Work out the finished part from the listing and answer in its coordinate system (mm). A direction names the side the tool comes from. Coordinates: 2 decimals unless noted, no trailing zeros. Order: outer loops, then holes, each group sorted by start corner. A loop starts at its lowest first (then second) coordinate and runs counter-clockwise, first axis right, second up.
1. Find the intervals of material crossed by probe 1 along X at (y, z) = (-26, 60); probe 2 along Z at (x, y) = (-82.5, -55.5); probe 3 along Y at (x, z) = (65.5, 79), in increasing order.
2. Determine the mould class of faces 1 (the flat face through (-13, -58, 88)), 2 (the cylindrical face through (-155.15, -47.633, 41.658)), 3 (the cylindrical face through (149.726, -44.75, 43.384)) for opening direction X: +X half, -X half, draft (parallel to the pull), parting line (faces both ways), or undercut.
3. A tool of negligible diameter and unlimited length cuts with its end or side. For faces 4 (the flat face through (-2, 2, -6)), 5 (the flat face through (-2, -58, 10)), 6 (the cylindrical face through (-150.2, -44.2, 43.4)), from which of +Z, -Z, +X, -X, +Y, -Y can it reach the whole face along a straight path? Write none if from no direction.
4. Flat-ended cylindrical pins translate along their axes: pin 1 Ø3 at (y, z) = (-57.5, 34) entering from -X; pin 2 Ø5 at (y, z) = (35, 49.5) entering from -X; pin 3 Ø3 at (y, z) = (-57, 53) entering from +X. Find the tip coordinate at first contact, or state that the pin passes through.
5. The part is cut by section A-A, the plane x = 71. Give the vertices of the cut face in (y, z).
6. The part is cut by section D-D, the plane y = 36. Give the vertices of the cut face in (x, z), then the cut area to 3 significant figures.
7. The part is cut by section C-C, the plane y = -30. Give the vertices of the cut face in (x, z).
8. The part is cut by section B-B, the plane z = 82.5. Give the vertices of the cut face in (x, y), then the cut area to 3 significant figures.
```python
from build123d import *

# Parameters (mm, degrees)
BOSS_EXTRUDE1_DEPTH = 88
SKETCH3_W           = 233.89900304
SKETCH3_H           = 68
CUT_EXTRUDE1_DEPTH  = 15
BOSS_EXTRUDE2_DEPTH = 6


with BuildPart() as part:
    # Sketch1 → Boss-Extrude1 (new body)
    with BuildSketch(Plane.XY):
        with BuildLine():
            Line((118.214818276, 64.136748505), (-118.214818276, 64.136748505))
            Line((-118.214818276, 64.136748505), (-162.822637659, -18.216148816))
            ThreePointArc((-162.822637659, -18.216148816), (-154.866072847, -47.976045164), (-126.94950152, -61))
            Line((-126.94950152, -61), (126.94950152, -61))
            ThreePointArc((126.94950152, -61), (154.866072847, -47.976045164), (162.822637659, -18.216148816))
            Line((162.822637659, -18.216148816), (118.214818276, 64.136748505))
        make_face()
        with BuildLine():
            Line((114.641146244, 58.136748505), (-114.641146244, 58.136748505))
            Line((-114.641146244, 58.136748505), (-157.062609578, -20.179799188))
            ThreePointArc((-157.062609578, -20.179799188), (-149.967134226, -44.474777247), (-126.94950152, -55))
            Line((-126.94950152, -55), (126.94950152, -55))
            ThreePointArc((126.94950152, -55), (149.967134226, -44.474777247), (157.062609578, -20.179799188))
            Line((157.062609578, -20.179799188), (114.641146244, 58.136748505))
        make_face(mode=Mode.SUBTRACT)
    extrude(amount=BOSS_EXTRUDE1_DEPTH)

    # Sketch3 → Cut-Extrude1 (cut)
    with BuildSketch(Plane.XZ.offset(46)):
        with Locations((0, 44)):
            Rectangle(SKETCH3_W, SKETCH3_H)
    extrude(amount=CUT_EXTRUDE1_DEPTH, mode=Mode.SUBTRACT)

    # Sketch1<12> → Boss-Extrude2 (add)
    with BuildSketch(Plane.XY):
        with BuildLine():
            Line((162.822637659, -18.216148816), (118.214818276, 64.136748505))
            Line((118.214818276, 64.136748505), (-118.214818276, 64.136748505))
            Line((-118.214818276, 64.136748505), (-162.822637659, -18.216148816))
            ThreePointArc((-162.822637659, -18.216148816), (-154.866072847, -47.976045164), (-126.94950152, -61))
            Line((-126.94950152, -61), (126.94950152, -61))
            ThreePointArc((126.94950152, -61), (154.866072847, -47.976045164), (162.822637659, -18.216148816))
        make_face()
    extrude(amount=-BOSS_EXTRUDE2_DEPTH)


solid = part.part
```
Geometry says:
1. probe 1: x = -163.35 to -157.35, 157.35 to 163.35
1. probe 2: z = -6 to 10, 78 to 88
1. probe 3: y = -61 to -55, 58.14 to 64.14
2. face 1: draft
2. face 2: -X half
2. face 3: undercut
3. face 4: -Z, +X, -X, +Y, -Y
3. face 5: -Y
3. face 6: +Z
4. pin 1: stops at x = -145.37
4. pin 2: stops at x = -135.35
4. pin 3: stops at x = 146.2
5. outline: (-61, -6) - (64.14, -6) - (64.14, 88) - (58.14, 88) - (58.14, 0) - (-55, 0) - (-55, 10) - (-61, 10) - close; (-61, 78) - (-55, 78) - (-55, 88) - (-61, 88) - close
6. outline: (-133.46, -6) - (133.46, -6) - (133.46, 88) - (126.63, 88) - (126.63, 0) - (-126.63, 0) - (-126.63, 88) - (-133.46, 88) - close
6. area: 2,800 mm2
7. outline: (-162.97, -6) - (162.97, -6) - (162.97, 88) - (156.89, 88) - (156.89, 0) - (-156.89, 0) - (-156.89, 88) - (-162.97, 88) - close
8. outline: (-162.82, -18.22) arc R36.43 ccw to (-126.95, -61) - (126.95, -61) arc R36.43 ccw to (162.82, -18.22) - (118.21, 64.14) - (-118.21, 64.14) - close; hole (-157.06, -20.18) arc R30.43 ccw to (-126.95, -55) - (126.95, -55) arc R30.43 ccw to (157.06, -20.18) - (114.64, 58.14) - (-114.64, 58.14) - close
8. area: 4,710 mm2
